from build123d import *

# Parameters (mm, degrees)
SKETCH1_W            = 25
SKETCH1_H            = 40
SKETCH1_W_2          = 22
SKETCH1_H_2          = 37
BOSS_EXTRUDE1_DEPTH  = 950
SKETCH3_W            = 25
SKETCH3_H            = 40
SKETCH3_W_2          = 22
SKETCH3_H_2          = 37
BOSS_EXTRUDE2_DEPTH  = 950
SKETCH4_W            = 25
SKETCH4_H            = 40
SKETCH4_W_2          = 22
SKETCH4_H_2          = 37
BOSS_EXTRUDE3_DEPTH  = 300
SKETCH5_W            = 25
SKETCH5_H            = 40
SKETCH5_W_2          = 22
SKETCH5_H_2          = 37
BOSS_EXTRUDE4_DEPTH  = 300
CUT_EXTRUDE1_DEPTH   = 300
CUT_EXTRUDE2_DEPTH   = 300
BOSS_EXTRUDE5_DEPTH  = 40
BOSS_EXTRUDE6_DEPTH  = 40
SKETCH10_W           = 25
SKETCH10_H           = 300
BOSS_EXTRUDE7_DEPTH  = 40
SKETCH12_W           = 25
SKETCH12_H           = 40
SKETCH12_W_2         = 22
SKETCH12_H_2         = 37
BOSS_EXTRUDE8_DEPTH  = 100
SKETCH14_W           = 25
SKETCH14_H           = 40
SKETCH14_W_2         = 22
SKETCH14_H_2         = 37
BOSS_EXTRUDE9_DEPTH  = 350
SKETCH15_W           = 25
SKETCH15_H           = 40
SKETCH15_W_2         = 22
SKETCH15_H_2         = 37
BOSS_EXTRUDE10_DEPTH = 300
BOSS_EXTRUDE11_DEPTH = 5
BOSS_EXTRUDE12_DEPTH = 20
SKETCH19_R           = 20
CUT_EXTRUDE3_DEPTH   = 20
SKETCH21_W           = 12.5
SKETCH21_H           = 60.024303072
SKETCH21_W_2         = 70.240967534
SKETCH21_H_2         = 12.5
SKETCH21_W_3         = 88.627521068
BOSS_EXTRUDE13_DEPTH = 100
BOSS_EXTRUDE14_DEPTH = 10
FILLET1_R            = 2
FILLET2_R            = 2
FILLET3_R            = 2
FILLET4_R            = 2
BOSS_EXTRUDE15_DEPTH = 40
BOSS_EXTRUDE16_DEPTH = 40
SWEEP1_START         = -14.984844988
SWEEP1_DEPTH         = 39.984844988
SWEEP1_2_DEPTH       = 1.5
SWEEP1_START_2       = 23.5
SWEEP1_3_DEPTH       = 1.5
SWEEP2_START         = -14.984844988
SWEEP2_DEPTH         = 39.984844988
SWEEP2_2_DEPTH       = 1.5
SWEEP2_START_2       = 23.5
SWEEP2_3_DEPTH       = 1.5


# Read off the part's stored shape, not the designer's step: Sweep1, Sweep2
with BuildPart() as part:
    # Sketch1 → Boss-Extrude1 (new body)
    with BuildSketch(Plane(origin=(0, 0, 0), x_dir=(0, 0, -1), z_dir=(1, 0, 0))):
        with Locations((12.5, -20)):
            Rectangle(SKETCH1_W, SKETCH1_H)
        with Locations((12.5, -20)):
            Rectangle(SKETCH1_W_2, SKETCH1_H_2, mode=Mode.SUBTRACT)
    extrude(amount=BOSS_EXTRUDE1_DEPTH)



with BuildPart() as body_2:
    # Sketch3 → Boss-Extrude2 (new body)
    with BuildSketch(Plane(origin=(950, 0, 0), x_dir=(0, 0, -1), z_dir=(1, 0, 0))):
        with Locations((337.5, -20)):
            Rectangle(SKETCH3_W, SKETCH3_H)
        with Locations((337.5, -20)):
            Rectangle(SKETCH3_W_2, SKETCH3_H_2, mode=Mode.SUBTRACT)
    extrude(amount=-BOSS_EXTRUDE2_DEPTH)


with BuildPart() as part_1:
    add(part.part)

    add(body_2.part)  # Boss-Extrude3 merges body 2
    # Sketch4 → Boss-Extrude3 (add)
    with BuildSketch(Plane.XY.offset(-325)):
        with Locations((937.5, -20)):
            Rectangle(SKETCH4_W, SKETCH4_H)
        with Locations((937.5, -20)):
            Rectangle(SKETCH4_W_2, SKETCH4_H_2, mode=Mode.SUBTRACT)
    extrude(amount=BOSS_EXTRUDE3_DEPTH)

    # Sketch5 → Boss-Extrude4 (add)
    with BuildSketch(Plane.XY.offset(-325)):
        with Locations((12.5, -20)):
            Rectangle(SKETCH5_W, SKETCH5_H)
        with Locations((12.5, -20)):
            Rectangle(SKETCH5_W_2, SKETCH5_H_2, mode=Mode.SUBTRACT)
    extrude(amount=BOSS_EXTRUDE4_DEPTH)

    # Sketch6 → Cut-Extrude1 (cut)
    with BuildSketch(Plane(origin=(0, 0, 0), x_dir=(1, 0, 0), z_dir=(0, 1, 0))):
        with BuildLine():
            Line((925, 0), (950, 0))
            Line((950, 0), (950, 25))
            ThreePointArc((950, 25), (942.67766953, 7.32233047), (925, 0))
        make_face()
    extrude(amount=-CUT_EXTRUDE1_DEPTH, mode=Mode.SUBTRACT)

    # Sketch7 → Cut-Extrude2 (cut)
    with BuildSketch(Plane(origin=(0, 0, 0), x_dir=(1, 0, 0), z_dir=(0, 1, 0))):
        with BuildLine():
            Line((950, 325), (950, 350))
            Line((950, 350), (925, 350))
            ThreePointArc((925, 350), (942.67766953, 342.67766953), (950, 325))
        make_face()
    extrude(amount=-CUT_EXTRUDE2_DEPTH, mode=Mode.SUBTRACT)

    # Sketch8 → Boss-Extrude5 (add)
    with BuildSketch(Plane(origin=(0, 0, 0), x_dir=(1, 0, 0), z_dir=(0, 1, 0))):
        with BuildLine():
            Line((910, 25), (925, 25))
            Line((925, 25), (925, 40))
            ThreePointArc((925, 40), (920.606601718, 29.393398282), (910, 25))
        make_face()
    extrude(amount=-BOSS_EXTRUDE5_DEPTH)

    # Sketch9 → Boss-Extrude6 (add)
    with BuildSketch(Plane(origin=(0, 0, 0), x_dir=(1, 0, 0), z_dir=(0, 1, 0))):
        with BuildLine():
            Line((925, 310), (925, 325))
            Line((925, 325), (910, 325))
            ThreePointArc((910, 325), (920.606601718, 320.606601718), (925, 310))
        make_face()
    extrude(amount=-BOSS_EXTRUDE6_DEPTH)

    # Sketch10 → Boss-Extrude7 (add)
    with BuildSketch(Plane(origin=(0, 0, 0), x_dir=(1, 0, 0), z_dir=(0, 1, 0))):
        with Locations((812.5, 175)):
            Rectangle(SKETCH10_W, SKETCH10_H)
    extrude(amount=-BOSS_EXTRUDE7_DEPTH)



with BuildPart() as body_2_2:
    # Sketch12 → Boss-Extrude8 (new body)
    with BuildSketch(Plane.XY):
        with Locations((737.631643114, -60)):
            Rectangle(SKETCH12_W, SKETCH12_H)
        with Locations((737.631643114, -60)):
            Rectangle(SKETCH12_W_2, SKETCH12_H_2, mode=Mode.SUBTRACT)
    extrude(amount=BOSS_EXTRUDE8_DEPTH)


with BuildPart() as part_2:
    add(part_1.part)

    add(body_2_2.part)  # Boss-Extrude9 merges body 2 2
    # Sketch14 → Boss-Extrude9 (add)
    with BuildSketch(Plane(origin=(0, 0, 0), x_dir=(-1, 0, 0), z_dir=(0, 0, -1))):
        with Locations((-737.631643114, -60)):
            Rectangle(SKETCH14_W, SKETCH14_H)
        with Locations((-737.631643114, -60)):
            Rectangle(SKETCH14_W_2, SKETCH14_H_2, mode=Mode.SUBTRACT)
    extrude(amount=BOSS_EXTRUDE9_DEPTH)

    # Sketch15 → Boss-Extrude10 (add)
    with BuildSketch(Plane.XY.offset(-325)):
        with Locations((637.631643114, -20)):
            Rectangle(SKETCH15_W, SKETCH15_H)
        with Locations((637.631643114, -20)):
            Rectangle(SKETCH15_W_2, SKETCH15_H_2, mode=Mode.SUBTRACT)
    extrude(amount=BOSS_EXTRUDE10_DEPTH)

    # Sketch16 → Boss-Extrude11 (add)
    with BuildSketch(Plane(origin=(0, 0, -350), x_dir=(-1, 0, 0), z_dir=(0, 0, -1))):
        Polygon((-20, -40), (-220, -40), (-180, -120), (-60, -120), align=None)
    boss_extrude11 = extrude(amount=-BOSS_EXTRUDE11_DEPTH)

    # Mirror1: Boss-Extrude11 across plane
    add(boss_extrude11.mirror(Plane.XY.offset(-175)))

    # Sketch18 → Boss-Extrude12 (add)
    with BuildSketch(Plane.XY.offset(-345)):
        Polygon((60, -115), (57.5, -115), (60, -120), (100, -120), (100, -115), align=None)
        Polygon((180, -115), (182.5, -115), (180, -120), (140, -120), (140, -115), align=None)
    boss_extrude12 = extrude(amount=BOSS_EXTRUDE12_DEPTH)

    # Sketch19 → Cut-Extrude3 (cut)
    with BuildSketch(Plane.XY.offset(-345)):
        with Locations((120, -120)):
            Circle(SKETCH19_R)
    cut_extrude3 = extrude(amount=-CUT_EXTRUDE3_DEPTH, mode=Mode.SUBTRACT)

    # Mirror2: Boss-Extrude12, Cut-Extrude3 across plane
    add(boss_extrude12.mirror(Plane.XY.offset(-175)))
    add(cut_extrude3.mirror(Plane.XY.offset(-175)), mode=Mode.SUBTRACT)

    # Sketch21 → Boss-Extrude13 (add)
    with BuildSketch(Plane(origin=(0, 0, 0), x_dir=(1, 0, 0), z_dir=(0, 1, 0))):
        with Locations((6.25, 175)):
            Rectangle(SKETCH21_W, SKETCH21_H)
        with Locations((180, 343.75)):
            Rectangle(SKETCH21_W_2, SKETCH21_H_2)
        with Locations((180, 6.25)):
            Rectangle(SKETCH21_W_3, SKETCH21_H_2)
    extrude(amount=BOSS_EXTRUDE13_DEPTH)

    # Sketch22 → Boss-Extrude14 (add)
    with BuildSketch(Plane(origin=(0, 0, 0), x_dir=(1, 0, 0), z_dir=(0, 1, 0))):
        Polygon((0, 320), (25, 320), (25, 295), (0, 295), (-14.984844988, 295), (-14.984844988, 320), align=None)
        Polygon((0, 318.5), (-13.484844988, 318.5), (-13.484844988, 296.5), (0, 296.5), (23.5, 296.5), (23.5, 318.5), align=None, mode=Mode.SUBTRACT)
    boss_extrude14 = extrude(amount=BOSS_EXTRUDE14_DEPTH)

    # Mirror3: Boss-Extrude14 across plane
    add(boss_extrude14.mirror(Plane.XY.offset(-175)))

    # Fillet1
    fillet1_edges = [part_2.edges().sort_by_distance(p)[0] for p in [
        (12.5, 0, -55),
    ]]
    fillet(fillet1_edges, radius=FILLET1_R)

    # Fillet2
    fillet2_edges = [part_2.edges().sort_by_distance(p)[0] for p in [
        (12.5, 0, -295),
    ]]
    fillet(fillet2_edges, radius=FILLET2_R)

    # Fillet3
    fillet3_edges = [part_2.edges().sort_by_distance(p)[0] for p in [
        (12.5, 0, -320),
    ]]
    fillet(fillet3_edges, radius=FILLET3_R)

    # Fillet4
    fillet4_edges = [part_2.edges().sort_by_distance(p)[0] for p in [
        (12.5, 0, -30),
    ]]
    fillet(fillet4_edges, radius=FILLET4_R)

    # Sketch23 → Boss-Extrude15 (add)
    with BuildSketch(Plane.XZ):
        Polygon((0, -31.5), (0, -30), (-14.984844988, -30), (-14.984844988, -55), (0, -55), (0, -53.5), (-13.484844988, -53.5), (-13.484844988, -31.5), align=None)
    extrude(amount=BOSS_EXTRUDE15_DEPTH)

    # Sketch24 → Boss-Extrude16 (add)
    with BuildSketch(Plane.XZ):
        Polygon((0, -296.5), (0, -295), (-14.984844988, -295), (-14.984844988, -320), (0, -320), (0, -318.5), (-13.484844988, -318.5), (-13.484844988, -296.5), align=None)
    extrude(amount=BOSS_EXTRUDE16_DEPTH)

    # Sweep1 outline → Sweep1 (add)
    with BuildSketch(Plane.YZ.offset(SWEEP1_START)):
        Polygon((10, -318.5), (10, -320), (450, -280), (450, -278.5), align=None)
        Polygon((10, -295), (10, -296.5), (450, -256.5), (450, -255), align=None)
    extrude(amount=SWEEP1_DEPTH)

    # Sweep1 2 outline → Sweep1 2 (add)
    with BuildSketch(Plane.YZ.offset(SWEEP1_START)):
        Polygon((10, -296.5), (10, -318.5), (450, -278.5), (450, -256.5), align=None)
    extrude(amount=SWEEP1_2_DEPTH)

    # Sweep1 3 outline → Sweep1 3 (add)
    with BuildSketch(Plane.YZ.offset(SWEEP1_START_2)):
        Polygon((10, -296.5), (10, -318.5), (450, -278.5), (450, -256.5), align=None)
    extrude(amount=SWEEP1_3_DEPTH)

    # Sweep2 outline → Sweep2 (add)
    with BuildSketch(Plane.YZ.offset(SWEEP2_START)):
        Polygon((10, -55), (450, -95), (450, -93.5), (10, -53.5), align=None)
        Polygon((10, -31.5), (450, -71.5), (450, -70), (10, -30), align=None)
    extrude(amount=SWEEP2_DEPTH)

    # Sweep2 2 outline → Sweep2 2 (add)
    with BuildSketch(Plane.YZ.offset(SWEEP2_START)):
        Polygon((10, -53.5), (450, -93.5), (450, -71.5), (10, -31.5), align=None)
    extrude(amount=SWEEP2_2_DEPTH)

    # Sweep2 3 outline → Sweep2 3 (add)
    with BuildSketch(Plane.YZ.offset(SWEEP2_START_2)):
        Polygon((10, -53.5), (450, -93.5), (450, -71.5), (10, -31.5), align=None)
    extrude(amount=SWEEP2_3_DEPTH)


solid = part_2.part
Here's how the part is built. I have some questions about the finished solid (model axes, mm). A direction names the side the tool comes from. Coordinates: 2 decimals unless noted, no trailing zeros. Order: outer loops, then holes, each group sorted by start corner. A loop starts at its lowest first (then second) coordinate and runs counter-clockwise, first axis right, second up. Notation, with made-up numbers: M -32.75,-35 L 17.25,-35 A23 ccw 17.25,-21 Z; hole C 6,48 d6. An arc over 180 degrees is marked long. Answer as CSV lines item,"result".
Item 1: On a 3-axis mill with a long thin cutter (end or side, diameter ignored), from which of +Z, -Z, +X, -X, +Y, -Y can I reach the whole of each face in a straight line? I mean faces 1 (the face through (121, -71, -5)), 2 (the face through (738, -41.5, -122)), 3 (the face through (468, -20, -23.5)), 4 (the face through (4.75, 233.08, -73.78)). Say none if no direction works.
Results found:
face 1,"-X"
face 2,"+Z, -Z"
face 3,"+X, -X"
face 4,"none"
Item 2: Imagine slicing it at C-C on x = 403. Write out the boundary of the cut face in (y, z).
Results found:
outline,"M -40,-350 L 0,-350 L 0,-325 L -40,-325 Z; M -40,-25 L 0,-25 L 0,0 L -40,0 Z; hole M -38.5,-348.5 L -1.5,-348.5 L -1.5,-326.5 L -38.5,-326.5 Z; hole M -38.5,-23.5 L -1.5,-23.5 L -1.5,-1.5 L -38.5,-1.5 Z"
Item 3: Imagine slicing it at D-D on z = -125. Give the number of separate pieces and of enclosed holes in the cut face, plus the area to 3 significant figures.
Results found:
separate pieces,"5"
enclosed holes,"4"
area,"1,740 mm2"
Item 4: We'd pull the mould along X, two halves only. Please class faces 5 (the face through (25, 131, -63)), 6 (the face through (0, -18, -24)), 7 (the face through (160, -120, -338)): +X half, -X half, draft (parallel to the pull), parting line (faces both ways), or undercut.
Results found:
face 5,"undercut"
face 6,"-X half"
face 7,"draft"
Item 5: If I drill on line 1 (X direction, y = -59, z = 44.5); line 2 (X direction, y = 358, z = -284), over which ranges is the centre line in solid material (lowest first)?
Results found:
line 1,"725.13 to 726.63, 748.63 to 750.13"
line 2,"-14.98 to -13.48, 23.5 to 25"
Item 6: For pin 1 (5 mm diameter, centred on y = 173.5, z = -287, fed in from +X); pin 2 (6.5 mm diameter, centred on x = 337.5, z = -10.5, fed in from -Y); pin 3 (14 mm diameter, centred on y = 49.5, z = -8.5, fed in from +X), each with a flat end and sliding along its axis, tell me the tip position at first contact or that it passes through.
Results found:
pin 1,"x = 25"
pin 2,"y = -40"
pin 3,"x = 224.31"
Item 7: Imagine slicing it at B-B on y = 80. Write out the boundary of the cut face in (x, z).
Results found:
outline,"M -14.98,-313.64 L 25,-313.64 L 25,-288.64 L -14.98,-288.64 Z; M -14.98,-61.36 L 25,-61.36 L 25,-36.36 L -14.98,-36.36 Z; M 0,-205.01 L 12.5,-205.01 L 12.5,-144.99 L 0,-144.99 Z; M 135.69,-12.5 L 224.31,-12.5 L 224.31,0 L 135.69,0 Z; M 144.88,-350 L 215.12,-350 L 215.12,-337.5 L 144.88,-337.5 Z; hole M -13.48,-312.14 L 23.5,-312.14 L 23.5,-290.14 L -13.48,-290.14 Z; hole M -13.48,-59.86 L 23.5,-59.86 L 23.5,-37.86 L -13.48,-37.86 Z"
Item 8: Imagine slicing it at A-A on x = 196. Write out the boundary of the cut face in (y, z), plus the area to 3 significant figures.
Results found:
outline,"M -88,-350 L 100,-350 L 100,-337.5 L 0,-337.5 L 0,-325 L -40,-325 L -40,-345 L -88,-345 Z; M -88,-5 L -40,-5 L -40,-25 L 0,-25 L 0,-12.5 L 100,-12.5 L 100,0 L -88,0 Z; hole M -38.5,-348.5 L -1.5,-348.5 L -1.5,-326.5 L -38.5,-326.5 Z; hole M -38.5,-23.5 L -1.5,-23.5 L -1.5,-1.5 L -38.5,-1.5 Z"
area,"3,350 mm2"
